The model under review builds one solid part; all positions refer to its coordinate system, in mm. Give positions to 0.01 mm unless a question says otherwise; leave off trailing zeros. Loops run counter-clockwise (first coordinate to the right, second up) from the corner with the lowest first, then second, coordinate; pieces in that order, holes last. Notation, with made-up numbers: M 54,-36 L 77,-36 A26 ccw 77,-4 Z; hole C 25.25,-31 d5. An arc over 180 degrees is marked long. One line per item, written item: value. Start each with the question number.
Q1. For pin 1 (3 mm diameter, centred on y = -287.5, z = -20, fed in from +X), flat-tipped, find the tip position at first contact; note if it passes through.
Q2. We need section B-B on z = -15.5. Write out the cut boundary in (x, y).
Q3. To check wall thickness, follow line 1 along Z through (x, y) = (2, -1540.5); line 2 along X through (y, z) = (-1413, 60); line 3 along X through (y, z) = (-1682, -38). State the ranges of each line that lie inside material, in increasing order. Write a range as from..to.
Q4. We need section A-A on y = -1063. Write out the cut boundary in (x, z), plus the area to 3 significant figures.
```python
from build123d import *

# Parameters (mm, degrees)
F1_DEPTH = 1865
F3_DEPTH = 125.001
F4_R     = 9
F5_DEPTH = 7.5


with BuildPart() as f1:
    # F0 (on Front) → F1 (new body)
    with BuildSketch(Plane.XZ):
        with BuildLine():
            Line((-25.16784, 62.5), (-25.16784, -62.5))
            Line((-25.16784, -62.5), (39.83216, -62.5))
            Line((39.83216, -62.5), (39.83216, -55))
            Line((39.83216, -55), (-12.46784, -55))
            ThreePointArc((-12.46784, -55), (-18.124695, -52.656854), (-20.46784, -47))
            Line((-20.46784, -47), (-20.46784, 47))
            ThreePointArc((-20.46784, 47), (-18.124695, 52.656854), (-12.46784, 55))
            Line((-12.46784, 55), (39.83216, 55))
            Line((39.83216, 55), (39.83216, 62.5))
            Line((39.83216, 62.5), (-25.16784, 62.5))
        make_face()
    extrude(amount=F1_DEPTH)

    # F2 (on face) → F3 (cut, through all)
    with BuildSketch(Plane.XY.offset(62.5)):
        Polygon((39.83216, -1800), (-25.16784, -1865), (39.83216, -1865), align=None)
        Polygon((39.83216, 0), (-25.16784, 0), (-25.16784, -65), align=None)
    extrude(amount=-F3_DEPTH, mode=Mode.SUBTRACT)

    # F4 (on face) → F5 (cut, through all)
    with BuildSketch(Plane.XY.offset(62.5)):
        with Locations((7.33216, -350)):
            Circle(F4_R)
        with Locations((7.33216, -452)):
            Circle(F4_R)
        with Locations((7.33216, -1515)):
            Circle(F4_R)
        with Locations((7.33216, -1413)):
            Circle(F4_R)
    extrude(amount=-F5_DEPTH, mode=Mode.SUBTRACT)


solid = f1.part
```
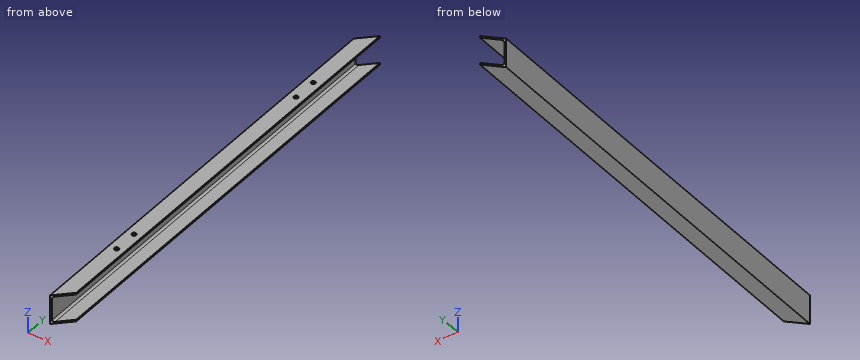
Solved:
1. pin 1: x = -20.47
2. outline: M -25.17,-1865 L -20.47,-1860.3 L -20.47,-60.3 L -25.17,-65 Z
3. line 1: -62.5..-55, 55..62.5
3. line 2: -25.17..-1.67, 16.33..39.83
3. line 3: -25.17..-20.47
4. outline: M -25.17,-62.5 L 39.83,-62.5 L 39.83,-55 L -12.47,-55 A8 cw -20.47,-47 L -20.47,47 A8 cw -12.47,55 L 39.83,55 L 39.83,62.5 L -25.17,62.5 Z
4. area: 1,520 mm2
